Can you work these out from the drawing? Everything is in mm from the part's minimum corner. A direction names the side the tool comes from. Round coordinates to 2 decimals unless told otherwise and drop trailing zeros. Write each loop counter-clockwise with the first axis right and the second up, starting at its lowest first coordinate (ties: lowest second). Pieces come first, ordered by that corner, then holes.
Q1. We'd pull the mould along X, two halves only. Please class the marked faces 3, 4 and 5: +X half, -X half, draft (parallel to the pull), parting line (faces both ways), or undercut.
Q2. I'm going to push a flat-ended pin straight in: pin 1 Ø5 at (x, z) = (21, 31.5) entering from +Y. Where does the tip first touch, or does it pass through?
Q3. If we section it at A-A (y = 16.25): Please give me the cut outline in (x, z), plus the area to 3 significant figures.
Q4. Please list where these lines run through material, in increasing order: line 1 along Z through (x, y) = (26, 9.5); line 2 along Z through (x, y) = (24, 11); line 3 along X through (y, z) = (8.5, 12).
Q5. If we section it at B-B (z = 36.5): Please give me the cut outline in (x, y).
Q6. For the marked faces 1 and 2, which set-ups out of +Z, -Z, +X, -X, +Y, -Y let a thin tool reach every point of the face, with its end or its side?
Q7. If we section it at C-C (x = 64): Please give me the cut outline in (y, z).
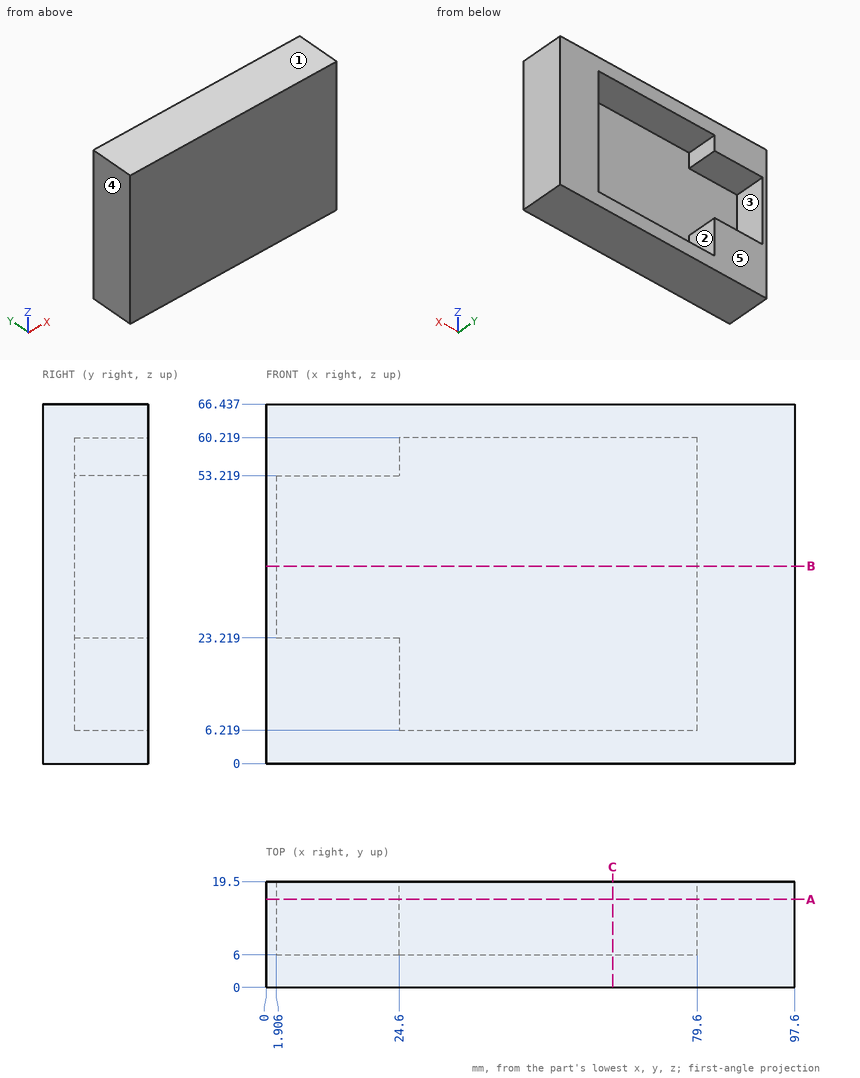
A:
1. face 3: undercut
1. face 4: -X half
1. face 5: draft
2. pin 1: stops at y = 6
3. outline: (0, 0) - (97.6, 0) - (97.6, 66.44) - (0, 66.44) - close; hole (1.91, 23.22) - (24.6, 23.22) - (24.6, 6.22) - (79.6, 6.22) - (79.6, 60.22) - (24.6, 60.22) - (24.6, 53.22) - (1.91, 53.22) - close
3. area: 2,830 mm2
4. line 1: z = 0 to 6.22, 60.22 to 66.44
4. line 2: z = 0 to 23.22, 53.22 to 66.44
4. line 3: x = 0 to 24.6, 79.6 to 97.6
5. outline: (0, 0) - (97.6, 0) - (97.6, 19.5) - (79.6, 19.5) - (79.6, 6) - (1.91, 6) - (1.91, 19.5) - (0, 19.5) - close
6. face 1: +Z, +X, -X, +Y, -Y
6. face 2: +Y
7. outline: (0, 0) - (19.5, 0) - (19.5, 6.22) - (6, 6.22) - (6, 60.22) - (19.5, 60.22) - (19.5, 66.44) - (0, 66.44) - close
